Here's the drawing with two shaded views (mm, measured from the low corner). I have some questions. Coordinates: 2 decimals unless noted, no trailing zeros. Write each loop counter-clockwise with the first axis right and the second up, starting at its lowest first coordinate (ties: lowest second). Pieces come first, ordered by that corner, then holes. Notation, with made-up numbers: (-39, 41) -> (18, 41) arc R23 cw to (18, 55) -> close; hole circle Ø9 at (32.5, 88). An arc over 180 degrees is marked (long way). Use one line per item in the form item = value.
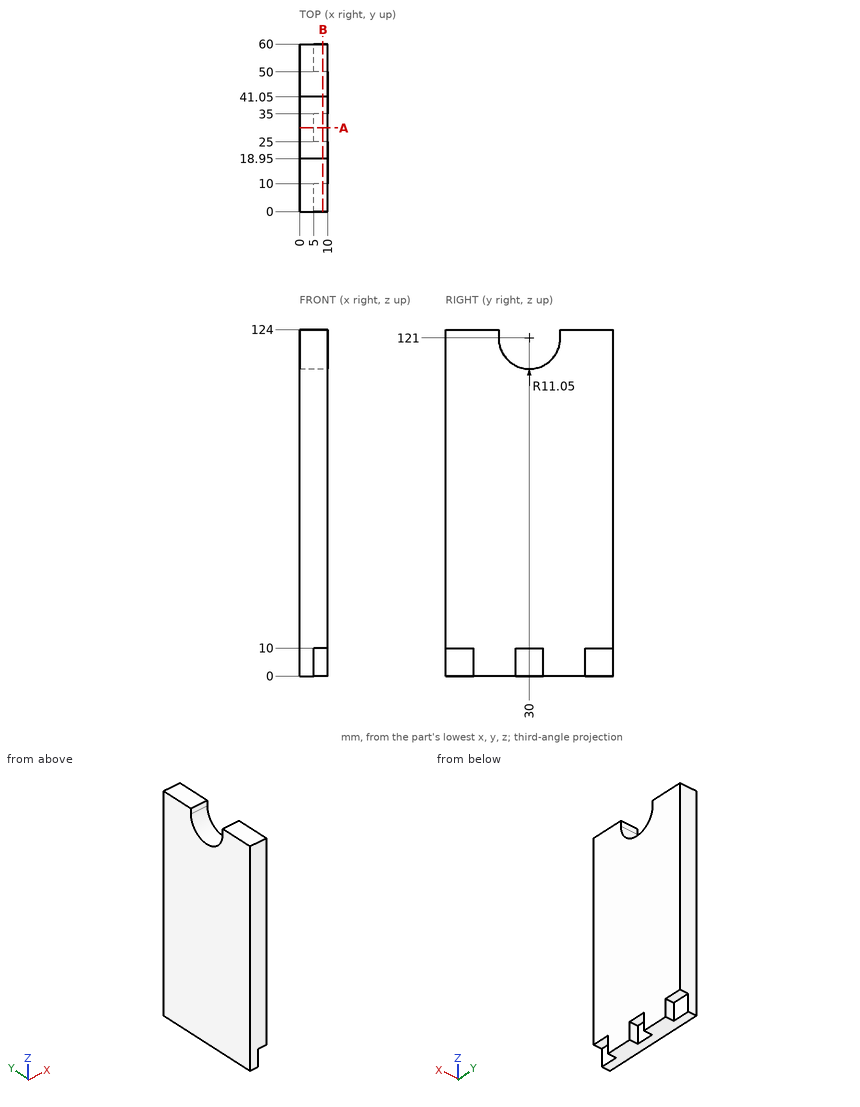
Q1. Suppose I cut it at B-B (x = 8.25). Write out the boundary of the cut face in (y, z), then the cut area to 3 significant figures.
Return value:
outline = (0, 10) -> (10, 10) -> (10, 0) -> (25, 0) -> (25, 10) -> (35, 10) -> (35, 0) -> (50, 0) -> (50, 10) -> (60, 10) -> (60, 124) -> (41.05, 124) -> (41.05, 121) arc R11.05 cw to (18.95, 121) -> (18.95, 124) -> (0, 124) -> close
area = 6,880 mm2
Q2. Will these pins go through, and if not, where does the flat tip stop? pin 1 (4 mm diameter, centred on x = 8, z = 2.5, fed in from +Y); pin 2 (4 mm diameter, centred on x = 8, z = 7.5, fed in from -Y); pin 3 (2.5 mm diameter, centred on x = 8.5, y = 57, fed in from -Z).
Return value:
pin_1 = 50
pin_2 = 10
pin_3 = 10
Q3. If I drill on line 1 (Z direction, x = 5.5, y = 53); line 2 (Z direction, x = 2.5, y = 22), over which ranges is the centre line in solid material (lowest first)? Write a range as from..to.
Return value:
line_1 = 10..124
line_2 = 0..113.38
Q4. Suppose I cut it at A-A (y = 30). Write out the boundary of the cut face in (x, z), then the cut area to 3 significant figures.
Return value:
outline = (0, 0) -> (5, 0) -> (5, 10) -> (10, 10) -> (10, 109.95) -> (0, 109.95) -> close
area = 1,050 mm2
